from build123d import *

# Parameters (mm, degrees)
EXTRUDE_SKETCH_1_R = 7.2
EXTRUDE_1_DEPTH    = 1.08
EXTRUDE_START      = 1.08
EXTRUDE_2_DEPTH    = 3.9
EXTRUDE_START_2    = -25
EXTRUDE_SKETCH_3_R = 3
EXTRUDE_3_DEPTH    = 25.01


with BuildPart() as part:
    # Extrude sketch 1 → Extrude 1 (new body)
    with BuildSketch(Plane.XY):
        Circle(EXTRUDE_SKETCH_1_R)
    extrude(amount=EXTRUDE_1_DEPTH)


with BuildPart() as body_2:
    # Extrude sketch 2 → Extrude 2 (new body)
    with BuildSketch(Plane.XY.offset(EXTRUDE_START)):
        Polygon((5, 2.886751346), (0, 5.773502692), (-5, 2.886751346), (-5, -2.886751346), (0, -5.773502692), (5, -2.886751346), align=None)
    extrude(amount=EXTRUDE_2_DEPTH)


with BuildPart() as body_3:
    # Extrude sketch 3 → Extrude 3 (new body)
    with BuildSketch(Plane.XY.offset(EXTRUDE_START_2)):
        Circle(EXTRUDE_SKETCH_3_R)
    extrude(amount=EXTRUDE_3_DEPTH)


with BuildPart() as body_2_1:
    add(body_2.part)

    # Combine (weld / assembly of features): union part, body 3
    add(part.part)
    add(body_3.part)


solid = body_2_1.part
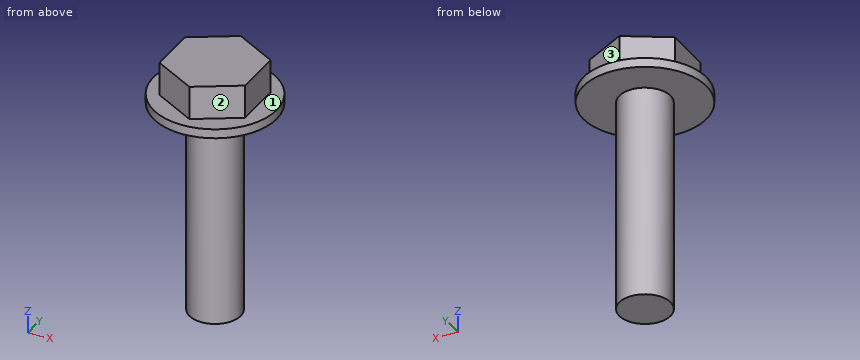
Check sheet for the modelled part. Datum: model origin and axes. Units: mm. Face numbers are marked on the shaded views. A direction names the side the tool comes from. Give positions to 0.01 mm unless a question says otherwise; leave off trailing zeros. Write each loop counter-clockwise with the first axis right and the second up, starting at its lowest first coordinate (ties: lowest second). Pieces come first, ordered by that corner, then holes. Notation, with made-up numbers: (-7, 23.5) -> (31, 23.5) arc R16 ccw to (31, 38.5) -> close; hole circle Ø4 at (73, 69). An arc over 180 degrees is marked (long way). Use one line per item in the form item = value. Start each with the question number.
1. Thickness scan on line 1 along Z through (x, y) = (3.25, -6); line 2 along Z through (x, y) = (3.5, 0.75); line 3 along X through (y, z) = (2.5, 2.5). Record the ranges inside material, lowest first. Write a range as from..to.
2. Section check A-A (y = 0). Record the cut outline in (x, z), and give its area (3 significant figures).
3. Section check C-C (x = 2). Record the cut outline in (y, z).
4. Access from +Z, -Z, +X, -X, +Y, -Y to the whole of each face (thin tool, end or side, straight path). Record for the marked faces 1, 2 and 3.
5. Section check B-B (z = 2.5). Record the cut outline in (x, y), and give its area (3 significant figures).
6. Section check D-D (y = 3.5). Record the cut outline in (x, z), and give its area (3 significant figures).
7. Go/stop test with flat-tipped pins: P1, Ø1.2, axis at y = -0.5, z = 2.5, coming from the -X side; P2, Ø6, axis at x = 5.5, y = 2.5, coming from the -Z side; P3, Ø1.2, axis at y = 1, z = 3.5, coming from the +X side. Record where each tip stops, or that it passes through.
Conclusion:
q1.line_1 = 0..1.08
q1.line_2 = 0..4.98
q1.line_3 = -5..5
q2.outline = (-7.2, 0) -> (-3, 0) -> (-3, -25) -> (3, -25) -> (3, 0) -> (7.2, 0) -> (7.2, 1.08) -> (5, 1.08) -> (5, 4.98) -> (-5, 4.98) -> (-5, 1.08) -> (-7.2, 1.08) -> close
q2.area = 205 mm²
q3.outline = (-6.92, 0) -> (-2.24, 0) -> (-2.24, -25) -> (2.24, -25) -> (2.24, 0) -> (6.92, 0) -> (6.92, 1.08) -> (4.62, 1.08) -> (4.62, 4.98) -> (-4.62, 4.98) -> (-4.62, 1.08) -> (-6.92, 1.08) -> close
q4.face_1 = +Z
q4.face_2 = +Z, +X, -Y
q4.face_3 = +Z, +X, +Y
q5.outline = (-5, -2.89) -> (0, -5.77) -> (5, -2.89) -> (5, 2.89) -> (0, 5.77) -> (-5, 2.89) -> close
q5.area = 86.6 mm²
q6.outline = (-6.29, 0) -> (6.29, 0) -> (6.29, 1.08) -> (3.94, 1.08) -> (3.94, 4.98) -> (-3.94, 4.98) -> (-3.94, 1.08) -> (-6.29, 1.08) -> close
q6.area = 44.3 mm²
q7.P1 = -5
q7.P2 = 0
q7.P3 = 5
